```python
from build123d import *

# Parameters (mm, degrees)
F0_W     = 15
F0_H     = 15
F1_DEPTH = 15
F2_W     = 12
F2_H     = 1.475
F3_DEPTH = 12
F4_R     = 5
F5_R     = 7
F6_DEPTH = 3.2
F7_SIZE2 = 3.19999
F7_SIZE  = 2.49999
F8_R     = 2.5
F9_SIZE  = 2


# Not quite as in the source:
# - a fillet or chamfer is up to 0.001 mm smaller than in the source, because OpenCascade refuses the exact size


with BuildPart() as f1:
    # F0 (on Top) → F1 (new body)
    with BuildSketch(Plane.XY):
        with Locations((7.5, 7.5)):
            Rectangle(F0_W, F0_H)
    extrude(amount=F1_DEPTH)

    # F2 (on face) → F3 (cut)
    with BuildSketch(Plane.XZ):
        with Locations((9, 12.2625)):
            Rectangle(F2_W, F2_H)
    extrude(amount=-F3_DEPTH, mode=Mode.SUBTRACT)

    # F4
    f4_edges = [f1.edges().sort_by_distance(p)[0] for p in [
        (3, 12, 12.2625),
    ]]
    fillet(f4_edges, radius=F4_R)

    # F5 (on face) → F6 (cut)
    with BuildSketch(Plane(origin=(0, 0, 0), x_dir=(1, 0, 0), z_dir=(0, 0, -1))):
        with Locations((7.5, -7.5)):
            Circle(F5_R)
    extrude(amount=-F6_DEPTH, mode=Mode.SUBTRACT)

    # F7 (size 2.5 and 3.2 in the source; OpenCascade refuses exactly that, so slightly less here)
    f7_edges = [f1.edges().sort_by_distance(p)[0] for p in [
        (0.5, 7.5, 3.2),
    ]]
    f7_side = f1.faces().sort_by_distance((7.5, 7.5, 3.2))[0]
    chamfer(f7_edges, length=F7_SIZE, length2=F7_SIZE2, reference=f7_side)

    # F8
    f8_edges = [f1.edges().sort_by_distance(p)[0] for p in [
        (15, 0, 14),
        (15, 0, 5.7625),
    ]]
    fillet(f8_edges, radius=F8_R)

    # F9
    f9_edges = [f1.edges().sort_by_distance(p)[0] for p in [
        (15, 15, 7.5),
        (0, 15, 7.5),
        (0, 0, 7.5),
    ]]
    chamfer(f9_edges, length=F9_SIZE)


solid = f1.part
```
Part model, mm, in its own coordinate system. A direction names the side the tool comes from. Coordinates: 2 decimals unless noted, no trailing zeros. Order: outer loops, then holes, each group sorted by start corner. A loop starts at its lowest first (then second) coordinate and runs counter-clockwise, first axis right, second up. Notation, with made-up numbers: (-4.5, 71.5) - (21.5, 71.5) arc R23 ccw to (21.5, 107.5) - close; hole circle Ø2 at (10.5, 63.25). An arc over 180 degrees is marked (long way). Return JSON: item names as keys, results as strings. Group by question number.
Item 1: Pin check, flat tips, straight feed: pin 1 (4 mm diameter, centred on x = 9.5, y = 11.5, fed in from -Z); pin 2 (6 mm diameter, centred on x = 9.5, y = 6, fed in from -Z); pin 3 (4.5 mm diameter, centred on x = 7, y = 5.5, fed in from -Z); pin 4 (4 mm diameter, centred on y = 2.5, z = 12, fed in from +X). Stop position of each tip, or through.
Item 2: Pull direction X, two halves, no side cores. Call faces 4 (the face through (9, 6, 13)), 5 (the face through (1, 1, 7)), 6 (the face through (3.8, 10.33, 3)): pulls with the +X half, pulls with the -X half, needs draft (parallel to the pull), parting line crosses it, or undercut.
Item 3: Drill centre lines: probe 1 along Z at (x, y) = (8, 7.25) (3 decimals); probe 2 along X at (y, z) = (4.5, 2.75); probe 3 along X at (y, z) = (7.5, 0.05). Where is each one in solid material? Low to high. Write a range as from..to.
Item 4: Which spindle directions (+Z, -Z, +X, -X, +Y, -Y) get a long thin tool onto all of the face, cutting with end or side? Do faces 1 (the face through (4, 10, 12)), 2 (the face through (14, 14, 7)), 3 (the face through (7, 7, 3.2)). Say none if no direction does.
Item 5: Cut at A-A (z = 14.25). List the corners of the cut face in (x, y).
Check values:
{
 "1": {"pin 1": "stops at z = 0.68", "pin 2": "stops at z = 1.92", "pin 3": "stops at z = 3.2", "pin 4": "stops at x = 15"},
 "2": {"face 4": "needs draft", "face 5": "pulls with the -X half", "face 6": "undercut"},
 "3": {"probe 1": "z = 3.2..11.525, 13..15", "probe 2": "x = 0..3.69, 11.31..15", "probe 3": "x = 0..0.54, 14.46..15"},
 "4": {"face 1": "+X, -Y", "face 2": "+Z, -Z, +X, +Y", "face 3": "-Z"},
 "5": {"outline": "(0, 2) - (2, 0) - (12.5, 0) arc R2.5 ccw to (15, 2.5) - (15, 13) - (13, 15) - (2, 15) - (0, 13) - close"}
}
